Geometry: see drawing. Coordinates: mm, zero at the bounding-box minimum. Give positions to 0.01 mm unless a question says otherwise; leave off trailing zeros. Loops run counter-clockwise (first coordinate to the right, second up) from the corner with the lowest first, then second, coordinate; pieces in that order, holes last. Notation, with made-up numbers: M -1,-2.75 L 12,-2.75 A11 ccw 12,11.25 Z; hole C 20,40.5 d6. An arc over 180 degrees is marked long. Use a Markdown table: item, result. Add a question column.
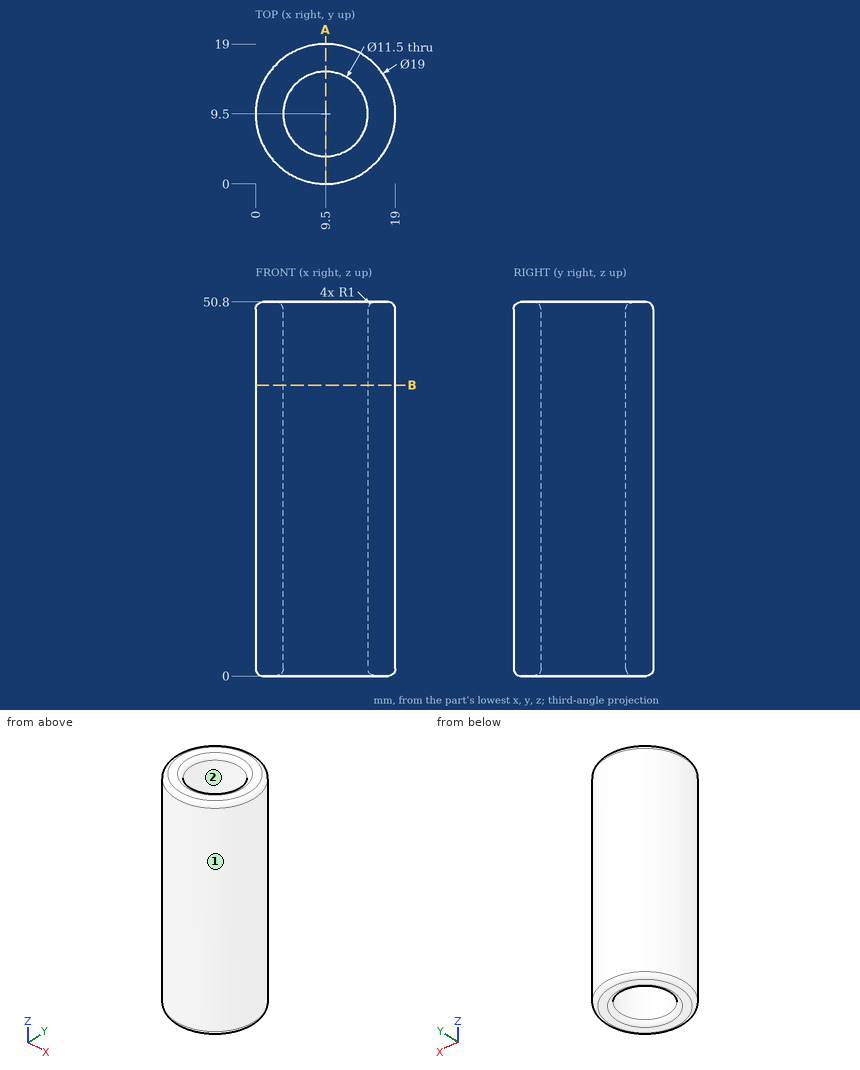
1) Pull-direction query (X, two-part tool) for the marked faces 1 and 2; classes: pulls with the +X half, pulls with the -X half, needs draft (parallel to the pull), parting line crosses it, or undercut.
2) Section query A-A, the plane x = 9.5. Return the cut outline in (y, z), and give its area (3 significant figures).
3) Ray query, line 1 (Y direction, x = 9.5, z = 21); line 2 (Y direction, x = 8, z = 6); line 3 (X direction, y = 14, z = 14). Return the intervals inside material, ascending. Write a range as [from, to].
4) Contact query for flat-ended pins moving along their axis: P1, Ø1, axis at y = 6, z = 45, coming from the -X side; P2, Ø5, axis at x = 5.5, z = 17, coming from the -Y side; P3, Ø1.5, axis at x = 8.5, z = 36.5, coming from the +Y side. Output: stop coordinate, or through.
5) Section query B-B, the plane z = 39.5. Return the cut outline in (x, y), and give its area (3 significant figures).
Entries:
| question | item | result |
|---|---|---|
| 1 | face 1 | parting line crosses it |
| 1 | face 2 | undercut |
| 2 | outline | M 0,1 A1 ccw 1,0 L 2.75,0 A1 ccw 3.75,1 L 3.75,49.8 A1 ccw 2.75,50.8 L 1,50.8 A1 ccw 0,49.8 Z; M 15.25,1 A1 ccw 16.25,0 L 18,0 A1 ccw 19,1 L 19,49.8 A1 ccw 18,50.8 L 16.25,50.8 A1 ccw 15.25,49.8 Z |
| 2 | area | 379 mm² |
| 3 | line 1 | y = [0, 3.75], [15.25, 19] |
| 3 | line 2 | y = [0.12, 3.95], [15.05, 18.88] |
| 3 | line 3 | x = [1.13, 5.92], [13.08, 17.87] |
| 4 | P1 | stops at x = 0.49 |
| 4 | P2 | stops at y = 0.12 |
| 4 | P3 | stops at y = 19 |
| 5 | outline | C 9.5,9.5 d19; hole C 9.5,9.5 d11.5 |
| 5 | area | 180 mm² |
